from build123d import *

# Parameters (mm, degrees)
SKETCH1_R           = 2.5
BOSS_EXTRUDE1_DEPTH = 10
CHAMFER1_SIZE       = 1
CHAMFER2_SIZE       = 0.5


with BuildPart() as part:
    # Sketch1 → Boss-Extrude1 (new body)
    # profile 1 of 2: a face of its own
    with BuildSketch(Plane(origin=(0, 0, 0), x_dir=(0, 1, 0), z_dir=(0, 0, 1))):
        with BuildLine():
            ThreePointArc((-3, 20), (-1.535533906, 23.535533906), (2, 25))
            Line((2, 25), (6, 25))
            ThreePointArc((6, 25), (9.535533906, 23.535533906), (11, 20))
            Line((11, 20), (11, 2))
            ThreePointArc((11, 2), (9.535533906, -1.535533906), (6, -3))
            Line((6, -3), (2, -3))
            ThreePointArc((2, -3), (-1.535533906, -1.535533906), (-3, 2))
            Line((-3, 2), (-3, 20))
        make_face()
        with BuildLine():
            Line((2, 22), (6, 22))
            ThreePointArc((6, 22), (7.414213562, 21.414213562), (8, 20))
            Line((8, 20), (8, 2))
            ThreePointArc((8, 2), (7.414213562, 0.585786438), (6, 0))
            Line((6, 0), (2, 0))
            ThreePointArc((2, 0), (0.585786438, 0.585786438), (0, 2))
            Line((0, 2), (0, 20))
            ThreePointArc((0, 20), (0.585786438, 21.414213562), (2, 22))
        make_face(mode=Mode.SUBTRACT)
    # profile 2 of 2: a face of its own
    with BuildSketch(Plane(origin=(0, 0, 0), x_dir=(0, 1, 0), z_dir=(0, 0, 1))):
        with BuildLine():
            Line((2, -13), (6, -13))
            ThreePointArc((6, -13), (9.535533906, -11.535533906), (11, -8))
            Line((11, -8), (11, 2))
            ThreePointArc((11, 2), (9.535533906, -1.535533906), (6, -3))
            Line((6, -3), (2, -3))
            ThreePointArc((2, -3), (-1.535533906, -1.535533906), (-3, 2))
            Line((-3, 2), (-3, -8))
            ThreePointArc((-3, -8), (-1.535533906, -11.535533906), (2, -13))
        make_face()
        with Locations(Location((4, -7, 0), (0, 0, 270))):
            Circle(SKETCH1_R, mode=Mode.SUBTRACT)
    extrude(amount=BOSS_EXTRUDE1_DEPTH)

    # Chamfer1
    chamfer1_edges = [part.edges().sort_by_distance(p)[0] for p in [
        (4.5, 4, 0),
        (4.5, 4, 10),
    ]]
    chamfer(chamfer1_edges, length=CHAMFER1_SIZE)

    # Chamfer2
    chamfer2_edges = [part.edges().sort_by_distance(p)[0] for p in [
        (11.535533906, -1.535533906, 10),
        (13, 4, 10),
        (-21.414213562, 0.585786438, 0),
        (-11, 0, 0),
        (-0.585786438, 0.585786438, 0),
        (0, 4, 0),
        (-0.585786438, 7.414213562, 0),
        (-11, 8, 0),
        (-21.414213562, 7.414213562, 0),
        (-22, 4, 0),
        (11.535533906, 9.535533906, 10),
        (-23.535533906, -1.535533906, 0),
        (-25, 4, 0),
        (-23.535533906, 9.535533906, 0),
        (-6, 11, 0),
        (11.535533906, 9.535533906, 0),
        (13, 4, 0),
        (11.535533906, -1.535533906, 0),
        (-6, -3, 0),
        (-6, 11, 10),
        (-23.535533906, 9.535533906, 10),
        (-25, 4, 10),
        (-23.535533906, -1.535533906, 10),
        (-22, 4, 10),
        (-21.414213562, 7.414213562, 10),
        (-11, 8, 10),
        (-0.585786438, 7.414213562, 10),
        (-6, -3, 10),
        (0, 4, 10),
        (-0.585786438, 0.585786438, 10),
        (-11, 0, 10),
        (-21.414213562, 0.585786438, 10),
    ]]
    chamfer(chamfer2_edges, length=CHAMFER2_SIZE)


solid = part.part
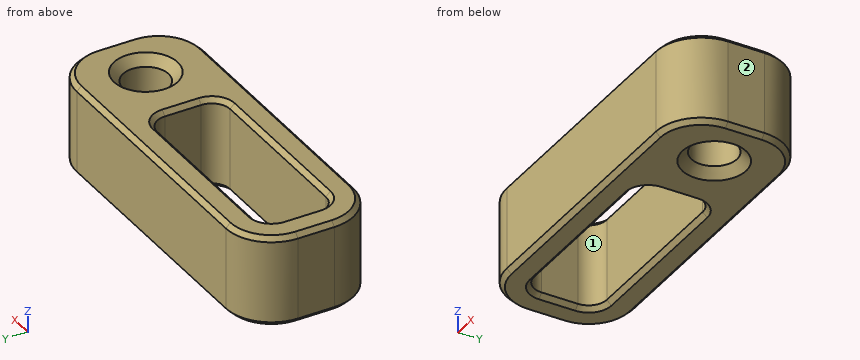
Verification items for the finished model (mm, model axes). Face numbers are marked on the shaded views. A direction names the side the tool comes from. Coordinates: 2 decimals unless noted, no trailing zeros. Loops run counter-clockwise (first coordinate to the right, second up) from the corner with the lowest first, then second, coordinate; pieces in that order, holes last. Notation, with made-up numbers: M 61.25,56.25 L 113.25,56.25 A10 ccw 113.25,75.25 Z; hole C -39.5,66.5 d4. An arc over 180 degrees is marked long. One line per item, written item: value.
1. Material ranges on line 1 along X through (y, z) = (5, 3); line 2 along Y through (x, z) = (7, 6.5); line 3 along Y through (x, z) = (-7.5, 1), recorded low to high. Write a range as from..to.
Answers follow:
line 1: -25..-22, 0..4.71, 9.29..13
line 2: -3..1.5, 6.5..11
line 3: -3..0, 8..11
2. Gauge pin test, flat ends, axial feed: P1, Ø8, axis at x = 7, y = 4, coming from the +Z side; P2, Ø1.5, axis at x = 8.5, y = 3.5, coming from the -Z side. Record the tip position at first contact, or that the pin passes through.
Answers follow:
P1: z = 10
P2: through
3. Section check A-A on x = 7. Record the cut outline in (y, z).
Answers follow:
outline: M -3,0.5 L -2.5,0 L 0.5,0 L 1.5,1 L 1.5,9 L 0.5,10 L -2.5,10 L -3,9.5 Z; M 6.5,1 L 7.5,0 L 10.5,0 L 11,0.5 L 11,9.5 L 10.5,10 L 7.5,10 L 6.5,9 Z
4. Section check C-C on z = 2.25. Record the cut outline in (x, y), plus the area to 3 significant figures.
Answers follow:
outline: M -25,2 A5 ccw -20,-3 L 8,-3 A5 ccw 13,2 L 13,6 A5 ccw 8,11 L -20,11 A5 ccw -25,6 Z; hole M -22,2 A2 ccw -20,0 L -2,0 A2 ccw 0,2 L 0,6 A2 ccw -2,8 L -20,8 A2 ccw -22,6 Z; hole C 7,4 d5
area: 318 mm^2
5. Section check B-B on y = 4. Record the cut outline in (x, z), plus the area to 3 significant figures.
Answers follow:
outline: M -25,0.5 L -24.5,0 L -22.5,0 L -22,0.5 L -22,9.5 L -22.5,10 L -24.5,10 L -25,9.5 Z; M 0,0.5 L 0.5,0 L 3.5,0 L 4.5,1 L 4.5,9 L 3.5,10 L 0.5,10 L 0,9.5 Z; M 9.5,1 L 10.5,0 L 12.5,0 L 13,0.5 L 13,9.5 L 12.5,10 L 10.5,10 L 9.5,9 Z
area: 107 mm^2
6. Set-up check for the marked faces 1 and 2: record each of +Z, -Z, +X, -X, +Y, -Y from which the full face is reachable in a straight line by a thin tool's end or side.
Answers follow:
face 1: +Z, -Z
face 2: +Z, -Z, +X, +Y, -Y
7. Section check D-D on x = -13.5. Record the cut outline in (y, z), plus the area to 3 significant figures.
Answers follow:
outline: M -3,0.5 L -2.5,0 L -0.5,0 L 0,0.5 L 0,9.5 L -0.5,10 L -2.5,10 L -3,9.5 Z; M 8,0.5 L 8.5,0 L 10.5,0 L 11,0.5 L 11,9.5 L 10.5,10 L 8.5,10 L 8,9.5 Z
area: 59.0 mm^2
